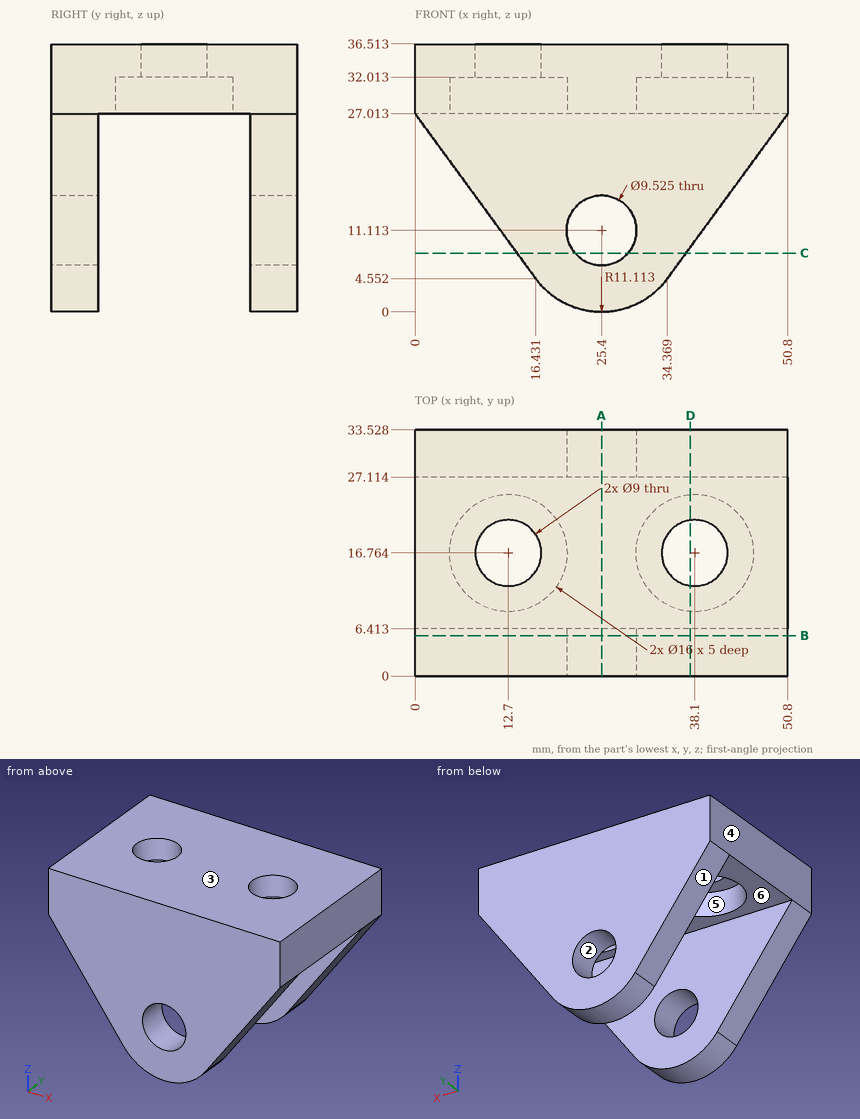
Could you check a few things on this drawing? It's one solid part, dimensions in mm from its lowest x, y, z. A direction names the side the tool comes from. Round coordinates to 2 decimals unless told otherwise and drop trailing zeros. Order: outer loops, then holes, each group sorted by start corner. A loop starts at its lowest first (then second) coordinate and runs counter-clockwise, first axis right, second up.
(1) Imagine slicing it at B-B (y = 5.5). Write out the boundary of the cut face in (x, z) (1 decimal), plus the area to 3 significant figures.
Response values:
outline: (0, 27) - (16.4, 4.6) arc R11.1 ccw to (34.4, 4.6) - (50.8, 27) - (50.8, 36.5) - (0, 36.5) - close; hole circle Ø9.5 at (25.4, 11.1)
area: 1,240 mm2
(2) Imagine slicing it at A-A (x = 25.4). Count the separate pieces of the cut face and the enclosed holes in it, plus the area to 3 significant figures.
Response values:
separate pieces: 3
enclosed holes: 0
area: 543 mm2
(3) Imagine slicing it at C-C (z = 8). Write out the boundary of the cut face in (x, y) (1 decimal).
Response values:
outline: (13.9, 0) - (21.8, 0) - (21.8, 6.4) - (13.9, 6.4) - close; (13.9, 27.1) - (21.8, 27.1) - (21.8, 33.5) - (13.9, 33.5) - close; (29, 0) - (36.9, 0) - (36.9, 6.4) - (29, 6.4) - close; (29, 27.1) - (36.9, 27.1) - (36.9, 33.5) - (29, 33.5) - close
(4) I'm going to push flat-ended pins straight in: pin 1 (13 mm diameter, centred on x = 15.5, y = 15.5, fed in from -Z); pin 2 (12 mm diameter, centred on x = 40.5, y = 25, fed in from -Z) (1 decimal); pin 3 (10 mm diameter, centred on x = 31.5, y = 11, fed in from -Z). Where does each tip first touch, or does it pass through?
Response values:
pin 1: stops at z = 27.01
pin 2: stops at z = 5.3
pin 3: stops at z = 0.79
(5) Please list where these lines run through material, in increasing order: line 1 along Y through (x, z) = (20, 19.5) (1 decimal); line 2 along Y through (x, z) = (38, 30) (1 decimal); line 3 along X through (y, z) = (22.5, 31.5) (1 decimal).
Response values:
line 1: y = 0 to 6.4, 27.1 to 33.5
line 2: y = 0 to 8.8, 24.8 to 33.5
line 3: x = 0 to 7.1, 18.3 to 32.5, 43.7 to 50.8
(6) If we mould it in two halves opening along X, with no side actions, what happens to the marked faces 1, 2 and 3? For each: released by +X, released by -X, zero draft, split by the parting line, or undercut.
Response values:
face 1: released by -X
face 2: undercut
face 3: zero draft
(7) Imagine slicing it at D-D (x = 37.5). Write out the boundary of the cut face in (y, z) (1 decimal), plus the area to 3 significant figures.
Response values:
outline: (0, 8.8) - (6.4, 8.8) - (6.4, 27) - (8.8, 27) - (8.8, 32) - (12.3, 32) - (12.3, 36.5) - (0, 36.5) - close; (21.2, 32) - (24.7, 32) - (24.7, 27) - (27.1, 27) - (27.1, 8.8) - (33.5, 8.8) - (33.5, 36.5) - (21.2, 36.5) - close
area: 432 mm2
(8) Which directions (+Z, -Z, +X, -X, +Y, -Y) give clear straight access to the entire face, cutting with the end or side of a thin tool? Please do the marked faces 4, 5 and 6.
Response values:
face 4: +Z, -Z, -X, +Y, -Y
face 5: -Z
face 6: -Z, +X, -X
